Build history of the part. All positions in model axes, mm. A direction names the side the tool comes from. Round coordinates to 2 decimals unless told otherwise and drop trailing zeros. Write each loop counter-clockwise with the first axis right and the second up, starting at its lowest first coordinate (ties: lowest second). Pieces come first, ordered by that corner, then holes. Notation, with made-up numbers: (39.5, -14.75) - (54.5, -14.75) arc R10 ccw to (54.5, -0.75) - close; hole circle Ø3 at (-11.5, 77.5). An arc over 180 degrees is marked (long way). Write each question's results on one line, items separated by ' | '.
from build123d import *

# Parameters (mm, degrees)
EXTRUDE_1_DEPTH     = 11
CUT_EXTRUDE_START   = -7
CUT_EXTRUDE_1_DEPTH = 7
SKETCH_3_R          = 2.05
CUT_EXTRUDE_2_DEPTH = 37
FILLET_1_R          = 2
EXTRUDE_START       = -4
EXTRUDE_2_DEPTH     = 4
SKETCH_5_W          = 34.461524683
SKETCH_5_H          = 8.345685775
CUT_EXTRUDE_3_DEPTH = 34
SKETCH_6_R          = 1.2
CUT_EXTRUDE_4_DEPTH = 10


with BuildPart() as part:
    # 草图1 → 凸台-拉伸1 (new body)
    with BuildSketch(Plane.XY):
        with BuildLine():
            Line((3.72790966, 78.977626184), (1, 78.977626184))
            ThreePointArc((1, 78.977626184), (0.292893219, 78.684732965), (0, 77.977626184))
            Line((0, 77.977626184), (0, -0.022373816))
            ThreePointArc((0, -0.022373816), (0.292893219, -0.729480597), (1, -1.022373816))
            Line((1, -1.022373816), (3.72790966, -1.022373816))
            ThreePointArc((3.72790966, -1.022373816), (4.801278091, -0.709940174), (5.539290113, 0.129745972))
            Line((5.539290113, 0.129745972), (13.303549433, 16.717027245))
            ThreePointArc((13.303549433, 16.717027245), (16.993609545, 20.915457973), (22.360451698, 22.477626184))
            Line((22.360451698, 22.477626184), (51.5, 22.477626184))
            ThreePointArc((51.5, 22.477626184), (52.560660172, 22.916966012), (53, 23.977626184))
            Line((53, 23.977626184), (53, 53.977626184))
            ThreePointArc((53, 53.977626184), (52.560660172, 55.038286356), (51.5, 55.477626184))
            Line((51.5, 55.477626184), (22.360451698, 55.477626184))
            ThreePointArc((22.360451698, 55.477626184), (16.993609545, 57.039794395), (13.303549433, 61.238225124))
            Line((13.303549433, 61.238225124), (5.539290113, 77.825506396))
            ThreePointArc((5.539290113, 77.825506396), (4.801278091, 78.665192542), (3.72790966, 78.977626184))
        make_face()
        with BuildLine():
            Line((46.723063893, 42.88691809), (40.887588257, 39.289675292))
            ThreePointArc((40.887588257, 39.289675292), (40.373853978, 38.759625352), (40.175145399, 38.048716955))
            ThreePointArc((40.175145399, 38.048716955), (40.339583189, 37.329108685), (40.827345936, 36.77506595))
            Line((40.827345936, 36.77506595), (46.483868127, 32.90251016))
            ThreePointArc((46.483868127, 32.90251016), (48.014920506, 32.805104134), (48.830807058, 34.104310989))
            Line((48.830807058, 34.104310989), (49.009760503, 41.574109577))
            ThreePointArc((49.009760503, 41.574109577), (48.257024254, 42.91089582), (46.723063893, 42.88691809))
        make_face(mode=Mode.SUBTRACT)
        with BuildLine():
            Line((35.975157614, 45.967771208), (23.29289503, 46.27159929))
            ThreePointArc((23.29289503, 46.27159929), (22.222016888, 45.857788357), (21.757400208, 44.807954643))
            ThreePointArc((21.757400208, 44.807954643), (21.945365563, 44.044228792), (22.493939434, 43.480602267))
            Line((22.493939434, 43.480602267), (28.780793319, 39.766059947))
            ThreePointArc((28.780793319, 39.766059947), (29.511034587, 39.557845657), (30.249678725, 39.733943182))
            Line((30.249678725, 39.733943182), (36.645087423, 43.144657419))
            ThreePointArc((36.645087423, 43.144657419), (37.398702379, 44.814536207), (35.975157614, 45.967771208))
        make_face(mode=Mode.SUBTRACT)
        with BuildLine():
            Line((28.711627706, 36.878978358), (22.254110192, 33.469752057))
            ThreePointArc((22.254110192, 33.469752057), (21.679175619, 32.933041346), (21.454853835, 32.179192628))
            ThreePointArc((21.454853835, 32.179192628), (21.868664769, 31.108314486), (22.918498482, 30.643697806))
            Line((22.918498482, 30.643697806), (35.600761065, 30.339869724))
            ThreePointArc((35.600761065, 30.339869724), (37.077896972, 31.42361332), (36.405111016, 33.127664295))
            Line((36.405111016, 33.127664295), (30.180365947, 36.840718678))
            ThreePointArc((30.180365947, 36.840718678), (29.451001862, 37.051985174), (28.711627706, 36.878978358))
        make_face(mode=Mode.SUBTRACT)
        with BuildLine():
            Line((8.398953615, 21.036666397), (15.693636896, 38.077972893))
            ThreePointArc((15.693636896, 38.077972893), (15.814233328, 38.63232963), (15.720321381, 39.191825329))
            Line((15.720321381, 39.191825329), (9.25005307, 56.562897813))
            ThreePointArc((9.25005307, 56.562897813), (7.596092236, 57.518632984), (6.344825548, 56.075252289))
            Line((6.344825548, 56.075252289), (5.520410579, 21.66287331))
            ThreePointArc((5.520410579, 21.66287331), (6.701123529, 20.161229848), (8.398953615, 21.036666397))
        make_face(mode=Mode.SUBTRACT)
    extrude(amount=EXTRUDE_1_DEPTH)

    # 草图2 → 切除-拉伸1 (cut)
    with BuildSketch(Plane.XY.offset(11).offset(CUT_EXTRUDE_START)):
        with BuildLine():
            Line((23, 22.477626184), (23, 27.477626184))
            Line((23, 27.477626184), (53, 27.477626184))
            Line((53, 27.477626184), (53, 50.477626184))
            Line((53, 50.477626184), (23, 50.477626184))
            Line((23, 50.477626184), (23, 55.477626184))
            Line((23, 55.477626184), (22.360451698, 55.477626184))
            ThreePointArc((22.360451698, 55.477626184), (16.993609545, 57.039794395), (13.303549433, 61.238225124))
            Line((13.303549433, 61.238225124), (5.539290113, 77.825506396))
            ThreePointArc((5.539290113, 77.825506396), (4.801278091, 78.665192542), (3.72790966, 78.977626184))
            Line((3.72790966, 78.977626184), (1, 78.977626184))
            ThreePointArc((1, 78.977626184), (0.292893219, 78.684732965), (0, 77.977626184))
            Line((0, 77.977626184), (0, -0.022373816))
            ThreePointArc((0, -0.022373816), (0.292893219, -0.729480597), (1, -1.022373816))
            Line((1, -1.022373816), (3.72790966, -1.022373816))
            ThreePointArc((3.72790966, -1.022373816), (4.801278091, -0.709940174), (5.539290113, 0.129745972))
            Line((5.539290113, 0.129745972), (13.303549433, 16.717027245))
            ThreePointArc((13.303549433, 16.717027245), (16.993609545, 20.915457973), (22.360451698, 22.477626184))
            Line((22.360451698, 22.477626184), (23, 22.477626184))
        make_face()
    extrude(amount=CUT_EXTRUDE_1_DEPTH, mode=Mode.SUBTRACT)

    # 草图3 → 切除-拉伸2 (cut)
    with BuildSketch(Plane(origin=(0, 55.477626184, 0), x_dir=(1, 0, 0), z_dir=(0, 1, 0))):
        with Locations(Location((48, -8, 0), (0, 0, 180))):
            Circle(SKETCH_3_R)
        with Locations(Location((28, -8, 0), (0, 0, 180))):
            Circle(SKETCH_3_R)
    extrude(amount=-CUT_EXTRUDE_2_DEPTH, mode=Mode.SUBTRACT)

    # 圆角1
    fillet_1_edges = [part.edges().sort_by_distance(p)[0] for p in [
        (53, 50.477626184, 7.5),
        (53, 27.477626184, 7.5),
        (23, 27.477626184, 7.5),
        (23, 22.477626184, 7.5),
        (23, 55.477626184, 7.5),
        (23, 50.477626184, 7.5),
    ]]
    fillet(fillet_1_edges, radius=FILLET_1_R)

    # 草图4 → 凸台-拉伸2 (add)
    with BuildSketch(Plane.XY.offset(4).offset(EXTRUDE_START)):
        with BuildLine():
            Line((5.935218909, 38.977626184), (15.782413333, 38.977626184))
            ThreePointArc((15.782413333, 38.977626184), (15.755353714, 39.08588132), (15.720321381, 39.191825329))
            Line((15.720321381, 39.191825329), (13.192788767, 45.977626184))
            Line((13.192788767, 45.977626184), (6.102917422, 45.977626184))
            Line((6.102917422, 45.977626184), (5.935218909, 38.977626184))
        make_face()
        with BuildLine():
            Line((5.767520396, 31.977626184), (13.082329062, 31.977626184))
            Line((13.082329062, 31.977626184), (15.693636896, 38.077972893))
            ThreePointArc((15.693636896, 38.077972893), (15.807413415, 38.520952405), (15.782413333, 38.977626184))
            Line((15.782413333, 38.977626184), (5.935218909, 38.977626184))
            Line((5.935218909, 38.977626184), (5.767520396, 31.977626184))
        make_face()
    extrude(amount=EXTRUDE_2_DEPTH)

    # 草图5 → 切除-拉伸3 (cut)
    with BuildSketch(Plane(origin=(0, 55.477626184, 0), x_dir=(1, 0, 0), z_dir=(0, 1, 0))):
        with Locations((40.230762341, -8.172842887)):
            Rectangle(SKETCH_5_W, SKETCH_5_H)
    extrude(amount=-CUT_EXTRUDE_3_DEPTH, mode=Mode.SUBTRACT)

    # 草图6 → 切除-拉伸4 (cut)
    with BuildSketch(Plane.XY.offset(4)):
        with Locations((38, 52.477626184)):
            Circle(SKETCH_6_R)
        with Locations((18, 52.477626184)):
            Circle(SKETCH_6_R)
        with Locations((18, 25.477626184)):
            Circle(SKETCH_6_R)
        with Locations((38, 25.477626184)):
            Circle(SKETCH_6_R)
    extrude(amount=-CUT_EXTRUDE_4_DEPTH, mode=Mode.SUBTRACT)


solid = part.part
(1) Slice it at C-C, the plane x = 45. Write the cut outline in (y, z).
Worked answers:
outline: (22.48, 0) - (33.92, 0) - (33.92, 4) - (22.48, 4) - close; (41.82, 0) - (55.48, 0) - (55.48, 4) - (41.82, 4) - close
(2) Flat gauge pins, fed straight in: pin 1 Ø2 at (x, z) = (9.5, 2) entering from +Y; pin 2 Ø2 at (x, z) = (33.5, 3) entering from +Y; pin 3 Ø2 at (x, z) = (9.5, 1.5) entering from -Y. Where does each tip first touch, or does it go through?
Worked answers:
pin 1: stops at y = 71.5 | pin 2: stops at y = 55.48 | pin 3: stops at y = 6.45
(3) Two-plate mould, pull along Y, no slides. Class faces 1 (the flat face through (20, 40, 4)), 2 (the cylindrical face through (39.1, 52, 2)), 3 (the cylindrical face through (4.81, 78.66, 1.97)): released by +Y, released by -Y, zero draft, split by the parting line, or undercut.
Worked answers:
face 1: zero draft | face 2: undercut | face 3: released by +Y
(4) Slice it at B-B, the plane y = 49.5. Write the cut outline in (x, z), and give its area (3 significant figures).
Worked answers:
outline: (0, 0) - (6.19, 0) - (6.19, 4) - (0, 4) - close; (11.88, 0) - (53, 0) - (53, 4) - (11.88, 4) - close | area: 189 mm2
(5) Slice it at A-A, the plane x = 32.5. Write the cut outline in (y, z), and give its area (3 significant figures).
Worked answers:
outline: (22.48, 0) - (30.41, 0) - (30.41, 4) - (22.48, 4) - close; (35.46, 0) - (40.93, 0) - (40.93, 4) - (35.46, 4) - close; (46.05, 0) - (55.48, 0) - (55.48, 4) - (46.05, 4) - close | area: 91.4 mm2
(6) Drill centre lines: probe 1 along Y at (x, z) = (38, 2.15); probe 2 along Y at (x, z) = (18, 2.5); probe 3 along X at (y, z) = (36.5, 1.15). Where is each one in solid material? Low to high. Write a range as [from, to].
Worked answers:
probe 1: y = [22.48, 24.28], [26.68, 51.28], [53.68, 55.48] | probe 2: y = [21.48, 24.28], [26.68, 51.28], [53.68, 56.48] | probe 3: x = [0, 27.99], [30.75, 41.23], [48.89, 53]
(7) Slice it at D-D, the plane z = 1.6. State how many separate pieces and enclosed holes the cut face has, and give its area (3 significant figures).
Worked answers:
separate pieces: 1 | enclosed holes: 9 | area: 1,920 mm2
(8) Tool access for faces 4 (the flat face through (10.708, 26.431, 1.972)), 5 (the cylindrical face through (17.06, 57, 1.97)): list every direction of +Z, -Z, +X, -X, +Y, -Y with a clear straight run to the whole face (end or side of a thin tool).
Worked answers:
face 4: +Z, -Z | face 5: +Z, -Z, +X, +Y
